```python
from build123d import *

# Parameters (mm, degrees)
SKETCH_1_R      = 11.75
SKETCH_1_R_2    = 9.25
EXTRUDE_1_DEPTH = 4
SKETCH_2_R      = 9.25
EXTRUDE_2_DEPTH = 4
CHAMFER_1_SIZE  = 0.5
FILLET_1_R      = 3


with BuildPart() as part:
    # 草图1 → 凸台-拉伸1 (new body)
    with BuildSketch(Plane(origin=(0, 0, 0), x_dir=(1, 0, 0), z_dir=(0, 1, 0))):
        with Locations(Location((0, 0, 0), (0, 0, 270))):
            Circle(SKETCH_1_R)
        with Locations(Location((0, 0, 0), (0, 0, 270))):
            Circle(SKETCH_1_R_2, mode=Mode.SUBTRACT)
    extrude(amount=EXTRUDE_1_DEPTH)

    # 草图2 → 凸台-拉伸2 (add)
    with BuildSketch(Plane(origin=(0, 4, 0), x_dir=(1, 0, 0), z_dir=(0, 1, 0))):
        Polygon((0, 11.75), (-10.175798494, 5.875), (-10.175798494, -5.875), (0, -11.75), (10.175798494, -5.875), (10.175798494, 5.875), align=None)
        with Locations(Location((0, 0, 0), (0, 0, 270))):
            Circle(SKETCH_2_R, mode=Mode.SUBTRACT)
    extrude(amount=EXTRUDE_2_DEPTH)

    # 倒角1
    chamfer_1_edges = [part.edges().sort_by_distance(p)[0] for p in [
        (5.087899247, 8, -8.8125),
        (-5.087899247, 8, -8.8125),
        (-10.175798494, 8, 0),
        (-5.087899247, 8, 8.8125),
        (5.087899247, 8, 8.8125),
        (10.175798494, 8, 0),
        (0, 0, -11.75),
    ]]
    chamfer(chamfer_1_edges, length=CHAMFER_1_SIZE)

    # 圆角1
    # the kernel refuses this fillet: 3 mm, written as the material it takes off along each edge
    with BuildSketch(Plane(origin=(-10.175798494, 4, 5.875), x_dir=(0.8660254037844421, 0, 0.49999999999999395), z_dir=(0, 1, 0)), Plane(origin=(-10.175798494, 4, -5.875), x_dir=(0, 0, 1), z_dir=(0, 1, 0)), Plane(origin=(0, 4, -11.75), x_dir=(-0.866025403784437, 0, 0.5000000000000027), z_dir=(0, 1, 0))) as fillet_1_piece_1:
        with BuildLine():
            CenterArc((FILLET_1_R * 0.57735026919, FILLET_1_R), FILLET_1_R, 210, 60)
            Line((-FILLET_1_R * 0.288675134595, FILLET_1_R * 0.5), (0, 0))
            Line((0, 0), (FILLET_1_R * 0.57735026919, 0))
        make_face()
    extrude(amount=7.830127019, mode=Mode.SUBTRACT)
    with BuildSketch(Plane(origin=(10.175798494, 4, -5.875), x_dir=(0, 0, 1), z_dir=(0, 1, 0)), Plane(origin=(10.175798494, 4, 5.875), x_dir=(-0.8660254037844379, 0, 0.5000000000000011), z_dir=(0, 1, 0)), Plane(origin=(0, 4, 11.75), x_dir=(-0.8660254037844418, 0, -0.4999999999999945), z_dir=(0, 1, 0))) as fillet_1_piece_2:
        with BuildLine():
            CenterArc((FILLET_1_R * 0.57735026919, -FILLET_1_R), FILLET_1_R, 90, 60)
            Line((-FILLET_1_R * 0.288675134595, -FILLET_1_R * 0.5), (0, 0))
            Line((0, 0), (FILLET_1_R * 0.57735026919, 0))
        make_face()
    extrude(amount=7.830127019, mode=Mode.SUBTRACT)
    with BuildSketch(Plane(origin=(7.820029772, 9.855768722, -4.514896294), x_dir=(0.2672612419124255, -0.2672612419124255, 0.9258200997725509), z_dir=(0.6546536707079768, -0.6546536707079768, -0.3779644730092288)), Plane(origin=(0, 9.855768722, 9.029792588), x_dir=(-0.935414346693487, -0.26726124191242306, -0.2314550249431329), z_dir=(3.5248488275713354e-15, -0.6546536707079781, 0.7559289460184537))) as fillet_1_piece_3:
        with BuildLine():
            CenterArc((FILLET_1_R * 0.377964473009, FILLET_1_R), FILLET_1_R, 228.590377891, 41.409622109)
            Line((-FILLET_1_R * 0.283473354757, FILLET_1_R * 0.25), (0, 0))
            Line((0, 0), (FILLET_1_R * 0.377964473009, 0))
        make_face()
    extrude(amount=6.433229711, mode=Mode.SUBTRACT)
    with BuildSketch(Plane(origin=(12.031567217, 5.644231278, 6.946428571), x_dir=(-0.66815310478106, -0.2672612419124238, 0.6943650748294146), z_dir=(-0.6546536707079774, 0.6546536707079774, -0.37796447300922653)), Plane(origin=(0, 9.855768722, -9.029792588), x_dir=(-0.935414346693485, -0.26726124191242234, 0.2314550249431414), z_dir=(-3.944473687996493e-15, -0.6546536707079779, -0.755928946018454)), Plane(origin=(-7.820029772, 9.855768722, -4.514896294), x_dir=(-0.26726124191242423, -0.26726124191242345, 0.9258200997725519), z_dir=(-0.6546536707079775, -0.6546536707079774, -0.37796447300922653)), Plane(origin=(-7.820029772, 9.855768722, 4.514896294), x_dir=(0.6681531047810633, -0.26726124191242634, 0.6943650748294108), z_dir=(-0.6546536707079768, -0.6546536707079768, 0.37796447300922886))) as fillet_1_piece_4:
        with BuildLine():
            CenterArc((FILLET_1_R * 0.377964473009, -FILLET_1_R), FILLET_1_R, 90, 41.409622109)
            Line((-FILLET_1_R * 0.283473354757, -FILLET_1_R * 0.25), (0, 0))
            Line((0, 0), (FILLET_1_R * 0.377964473009, 0))
        make_face()
    extrude(amount=6.433229711, mode=Mode.SUBTRACT)


solid = part.part
```
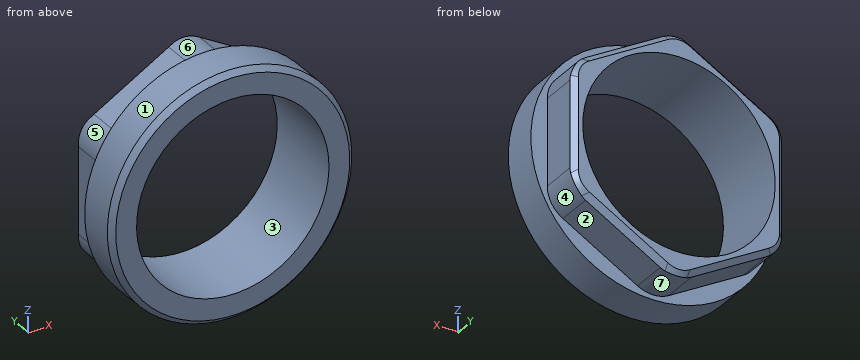
Model file for the job. Use its own axes, mm. Face numbers are marked on the shaded views. A direction names the side the tool comes from. Coordinates: 2 decimals unless noted, no trailing zeros. Write each loop counter-clockwise with the first axis right and the second up, starting at its lowest first coordinate (ties: lowest second). Pieces come first, ordered by that corner, then holes. Notation, with made-up numbers: (55.25, -24) - (70.25, -24) arc R24 cw to (70.25, 9) - close; hole circle Ø11 at (-8.5, -33). An arc over 180 degrees is marked (long way). Use a Markdown table: item, result. Add a question column.
Item 1: Two-plate mould, pull along Z, no slides. Class the marked faces 1, 2 and 3: pulls with the +Z half, pulls with the -Z half, needs draft (parallel to the pull), parting line crosses it, or undercut.
Item 2: Band-saw the part on A-A, the plane x = 0. Write the cut outline in (y, z).
Item 3: Band-saw the part on D-D, the plane y = 2.25. Write the cut outline in (x, z).
Item 4: Band-saw the part on C-C, the plane z = 0. Write the cut outline in (x, y).
Item 5: Drop flat-ended pins along their axis: pin 1 (12 mm diameter, centred on x = -3.5, z = -5.5, fed in from +Y); pin 2 (1 mm diameter, centred on y = 6.5, z = -2, fed in from -X); pin 3 (4 mm diameter, centred on y = 6.5, z = 1, fed in from +X). Give the stop position or say it passes through.
Item 6: Band-saw the part on B-B, the plane y = 5.5. Write the cut outline in (x, z).
Item 7: 3-axis set-ups, long thin cutter, end or side, ignore diameter. For the marked faces 4, 5, 6 and 7: which of +Z, -Z, +X, -X, +Y, -Y reach the whole face in a straight line?
Item 8: Drill centre lines: line 1 along X through (y, z) = (2.5, 0); line 2 along X through (y, z) = (6, 0); line 3 along Z through (x, y) = (-0.75, 2.5). Where is each one in solid material? Low to high.
A:
| question | item | result |
|---|---|---|
| 1 | face 1 | parting line crosses it |
| 1 | face 2 | pulls with the -Z half |
| 1 | face 3 | undercut |
| 2 | outline | (0, -11.25) - (0.5, -11.75) - (4, -11.75) - (4, -11.29) - (7.63, -11.29) - (8, -10.86) - (8, -9.25) - (0, -9.25) - close; (0, 9.25) - (8, 9.25) - (8, 10.86) - (7.63, 11.29) - (4, 11.29) - (4, 11.75) - (0.5, 11.75) - (0, 11.25) - close |
| 3 | outline | circle Ø23.5 at (0, 0); hole circle Ø18.5 at (0, 0) |
| 4 | outline | (-11.75, 0.5) - (-11.25, 0) - (-9.25, 0) - (-9.25, 8) - (-9.68, 8) - (-10.18, 7.5) - (-10.18, 4) - (-11.75, 4) - close; (9.25, 0) - (11.25, 0) - (11.75, 0.5) - (11.75, 4) - (10.18, 4) - (10.18, 7.5) - (9.68, 8) - (9.25, 8) - close |
| 5 | pin 1 | stops at y = 8 |
| 5 | pin 2 | stops at x = -10.18 |
| 5 | pin 3 | stops at x = 10.18 |
| 6 | outline | (-10.18, -4.14) arc R3 ccw to (-8.68, -6.74) - (-1.5, -10.88) arc R3 ccw to (1.5, -10.88) - (8.68, -6.74) arc R3 ccw to (10.18, -4.14) - (10.18, 4.14) arc R3 ccw to (8.68, 6.74) - (1.5, 10.88) arc R3 ccw to (-1.5, 10.88) - (-8.68, 6.74) arc R3 ccw to (-10.18, 4.14) - close; hole circle Ø18.5 at (0, 0) |
| 7 | face 4 | -Z, +X, +Y |
| 7 | face 5 | +Z, -X, +Y |
| 7 | face 6 | +Z, +Y |
| 7 | face 7 | -Z, +Y |
| 8 | line 1 | x = -11.75 to -9.25, 9.25 to 11.75 |
| 8 | line 2 | x = -10.18 to -9.25, 9.25 to 10.18 |
| 8 | line 3 | z = -11.73 to -9.22, 9.22 to 11.73 |
